```python
from build123d import *

# Parameters (mm, degrees)
SKETCH_1_W          = 56
SKETCH_1_H          = 110
EXTRUDE_1_DEPTH     = 40
SKETCH_3_W          = 56
SKETCH_3_H          = 72
EXTRUDE_2_DEPTH     = 40
SKETCH_4_R          = 36
SKETCH_4_R_2        = 24
EXTRUDE_3_DEPTH     = 25
SKETCH_5_R          = 30
SKETCH_5_R_2        = 24
EXTRUDE_4_DEPTH     = 5
CHAMFER_1_SIZE      = 40
FILLET_1_R          = 2
SKETCH_6_R          = 19.352
CUT_EXTRUDE_1_DEPTH = 147
CHAMFER_2_SIZE      = 1.648
SKETCH_7_R          = 30
SKETCH_7_R_2        = 24
EXTRUDE_5_DEPTH     = 9
SKETCH_8_R          = 2.05
CUT_EXTRUDE_2_DEPTH = 37


with BuildPart() as part:
    # Эскиз1 → Бобышка-Вытянуть1 (new body)
    with BuildSketch(Plane.XY):
        Rectangle(SKETCH_1_W, SKETCH_1_H)
    extrude(amount=EXTRUDE_1_DEPTH)

    # Эскиз3 → Бобышка-Вытянуть2 (add)
    with BuildSketch(Plane.XY.offset(40)):
        Rectangle(SKETCH_3_W, SKETCH_3_H)
        with BuildLine():
            Line((28, 36), (28, -36))
            Line((28, -36), (82, -36))
            ThreePointArc((82, -36), (46, 0), (82, 36))
            Line((82, 36), (28, 36))
        make_face()
        with BuildLine():
            ThreePointArc((82, 36), (46, 0), (82, -36))
            Line((82, -36), (82, -24))
            ThreePointArc((82, -24), (58, 0), (82, 24))
            Line((82, 24), (82, 36))
        make_face()
        with BuildLine():
            Line((82, -24), (82, -36))
            ThreePointArc((82, -36), (107.455844, -25.455844), (118, 0))
            ThreePointArc((118, 0), (107.455844, 25.455844), (82, 36))
            Line((82, 36), (82, 24))
            ThreePointArc((82, 24), (98.970563, 16.970563), (106, 0))
            ThreePointArc((106, 0), (98.970563, -16.970563), (82, -24))
        make_face()
    extrude(amount=EXTRUDE_2_DEPTH)

    # Эскиз4 → Бобышка-Вытянуть3 (add, symmetric)
    with BuildSketch(Plane.XY.offset(60)):
        with Locations((82, 0)):
            Circle(SKETCH_4_R)
        with Locations((82, 0)):
            Circle(SKETCH_4_R_2, mode=Mode.SUBTRACT)
    extrude(amount=EXTRUDE_3_DEPTH, both=True)

    # Эскиз5 → Бобышка-Вытянуть4 (add)
    with BuildSketch(Plane.XY.offset(85)):
        with Locations((82, 0)):
            Circle(SKETCH_5_R)
        with Locations((82, 0)):
            Circle(SKETCH_5_R_2, mode=Mode.SUBTRACT)
    extrude(amount=EXTRUDE_4_DEPTH)

    # Фаска1
    chamfer_1_edges = [part.edges().sort_by_distance(p)[0] for p in [
        (-28, 0, 80),
    ]]
    chamfer(chamfer_1_edges, length=CHAMFER_1_SIZE)

    # Скругление1
    fillet_1_edges = [part.edges().sort_by_distance(p)[0] for p in [
        (28, 0, 40),
    ]]
    fillet(fillet_1_edges, radius=FILLET_1_R)

    # Зеркальное отражение1: part across plane


with BuildPart() as part_1:
    add(part.part)
    add(part.part.mirror(Plane(origin=(0, 0, 0), x_dir=(1, 0, 0), z_dir=(0, 0, -1))))

    # Эскиз6 → Вырез-Вытянуть1 (cut, through all)
    with BuildSketch(Plane.ZY.offset(28)):
        Circle(SKETCH_6_R)
    extrude(amount=-CUT_EXTRUDE_1_DEPTH, mode=Mode.SUBTRACT)

    # Фаска2
    chamfer_2_edges = [part_1.edges().sort_by_distance(p)[0] for p in [
        (28, -13.68393, 13.68393),
        (-28, 13.68393, 13.68393),
    ]]
    chamfer(chamfer_2_edges, length=CHAMFER_2_SIZE)

    # Эскиз7 → Бобышка-Вытянуть5 (add)
    with BuildSketch(Plane.XY.offset(90)):
        with Locations((82, 0)):
            Circle(SKETCH_7_R)
        with Locations((82, 0)):
            Circle(SKETCH_7_R_2, mode=Mode.SUBTRACT)
    extrude(amount=EXTRUDE_5_DEPTH)

    # Эскиз8 → Вырез-Вытянуть2 (cut, through all)
    with BuildSketch(Plane(origin=(82, 0, 0), x_dir=(0, 0, -1), z_dir=(1, 0, 0))):
        with Locations((-92, 0)):
            Circle(SKETCH_8_R)
    extrude(amount=CUT_EXTRUDE_2_DEPTH, mode=Mode.SUBTRACT)


solid = part_1.part
```
Part model, mm, in its own coordinate system. A direction names the side the tool comes from. Round coordinates to 2 decimals unless told otherwise and drop trailing zeros. Loops run counter-clockwise (first coordinate to the right, second up) from the corner with the lowest first, then second, coordinate; pieces in that order, holes last.
Item 1: 3-axis set-ups, long thin cutter, end or side, ignore diameter. For faces 1 (the face through (31, 1, -80)), 2 (the face through (0, -45, 40)), 3 (the face through (0, 46, 40)): which of +Z, -Z, +X, -X, +Y, -Y reach the whole face in a straight line?
Item 2: Drill centre lines: line 1 (Z direction, x = 107, y = 0); line 2 (Z direction, x = 43.5, y = 5); line 3 (Y direction, x = 82, z = -49). Where is each one in solid material? Low to high.
Item 3: Cut at A-A, the plane x = 38.5. Give the cut face in (y, z), then the cut area to 3 significant figures.
Item 4: Mould opens along Y. For faces 4 (the face through (52.03, 1.32, 91.9)), 5 (the face through (68, 27, -85)), 6 (the face through (-26.5, -17.3, 9)) say: +Y half, -Y half, draft (parallel to the pull), parting line (faces both ways), or undercut.
Item 5: Cut at C-C, the plane z = 0. Give the cut face in (x, y).
Item 6: Drop flat-ended pins along their axis: P1, Ø12, axis at x = -8, z = 61, coming from the -Y side; P2, Ø12.5, axis at x = 9.5, z = -66, coming from the +Y side; P3, Ø12, axis at y = 43, z = -45, coming from the +X side. Give the stop position or say it passes through.
Item 7: Cut at D-D, the plane x = -0.5. Give the cut face in (y, z), then the cut area to 3 significant figures.
Item 8: Cut at B-B, the plane z = 73. Give the cut face in (x, y).
A:
1. face 1: -Z, -X
1. face 2: +Z, +X, -X, -Y
1. face 3: +Z, +X, -X, +Y
2. line 1: z = -90 to -35, 35 to 89.95, 94.05 to 99
2. line 2: z = -80 to -40, 40 to 80
2. line 3: y = -36 to -24, 24 to 36
3. outline: (-36, -80) - (36, -80) - (36, -40) - (-36, -40) - close; (-36, 40) - (36, 40) - (36, 80) - (-36, 80) - close
3. area: 5,760 mm2
4. face 4: parting line
4. face 5: draft
4. face 6: undercut
5. outline: (-28, -55) - (28, -55) - (28, -21) - (26.35, -19.35) - (-26.35, -19.35) - (-28, -21) - close; (-28, 21) - (-26.35, 19.35) - (26.35, 19.35) - (28, 21) - (28, 55) - (-28, 55) - close
6. P1: stops at y = -36
6. P2: stops at y = 36
6. P3: stops at x = 28
7. outline: (-55, -40) - (-36, -40) - (-36, -67.5) - (36, -67.5) - (36, -40) - (55, -40) - (55, 40) - (36, 40) - (36, 67.5) - (-36, 67.5) - (-36, 40) - (-55, 40) - close; hole circle Ø38.7 at (0, 0)
7. area: 11,600 mm2
8. outline: (5, -36) - (82, -36) arc R36 ccw to (82, 36) - (5, 36) - close; hole (82, 24) arc R24 ccw (long way) to (106, 0) arc R24 ccw to start
